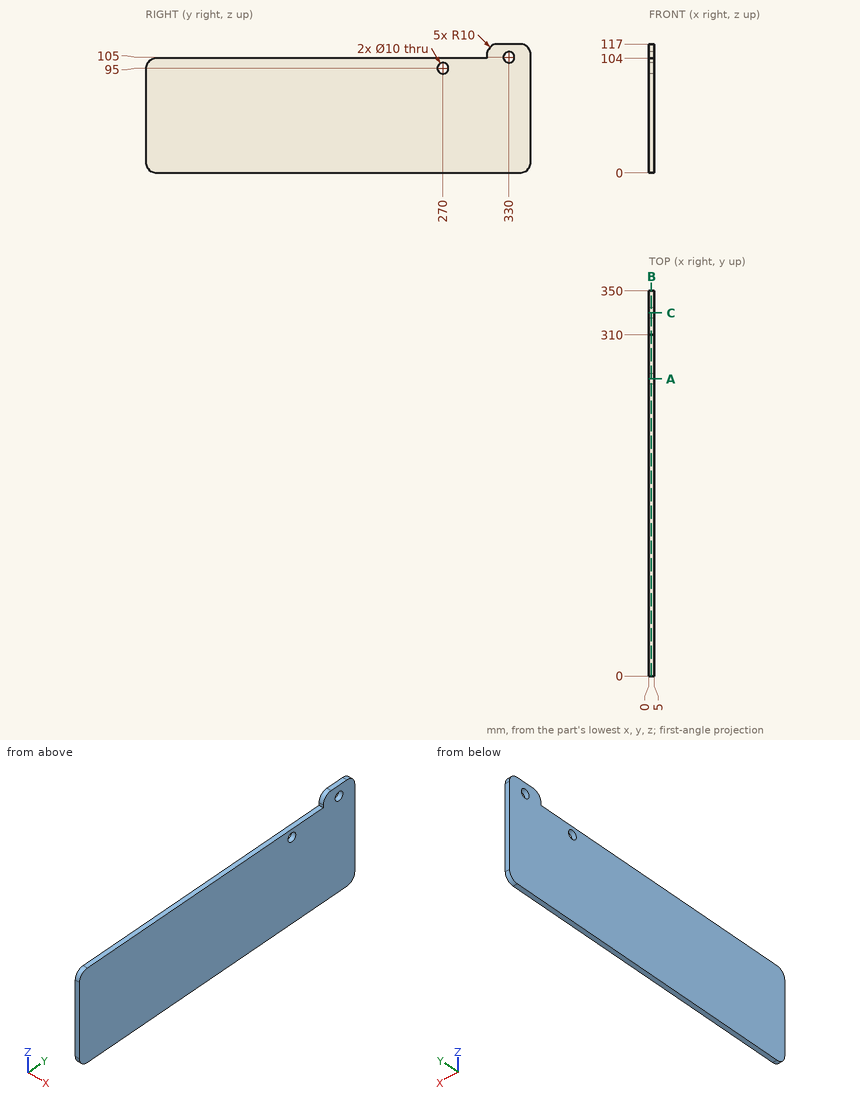
The drawing under review shows one solid part. Ordinate dimensions are in mm from its lowest x, y, z. Give positions to 0.01 mm unless a question says otherwise; leave off trailing zeros. Order: outer loops, then holes, each group sorted by start corner. A loop starts at its lowest first (then second) coordinate and runs counter-clockwise, first axis right, second up. Notation, with made-up numbers: M 37,-9 L 57,-9 A31 ccw 57,20 Z; hole C 50,-25.5 d2. An arc over 180 degrees is marked long. Answer in a Markdown table with one row per item. Add a question column.
1. Add section B-B on x = 2.25. State the section outline as (y, z) points.
2. To check wall thickness, follow line 1 along Z through (x, y) = (3.95, 330); line 2 along Z through (x, y) = (2.7, 173); line 3 along Y through (x, z) = (3.5, 102.5). State the ranges of each line that lie inside material, in increasing order.
3. Add section A-A on y = 270. State the section outline as (x, z) points, plus the area to 3 significant figures.
4. For pin 1 Ø2 at (x, y) = (4, 246) entering from +Z; pin 2 Ø2.5 at (x, z) = (3.5, 105.5) entering from -Y, all flat-tipped, find the tip position at first contact; note any pin that passes through.
5. Add section C-C on y = 330. State the section outline as (x, z) points, plus the area to 3 significant figures.
The answers:
| question | item | result |
|---|---|---|
| 1 | outline | M 0,10 A10 ccw 10,0 L 340,0 A10 ccw 350,10 L 350,107 A10 ccw 340,117 L 320,117 A10 ccw 310,107 L 310,104 L 10,104 A10 ccw 0,94 Z; hole C 270,95 d10; hole C 330,105 d10 |
| 2 | line 1 | 0 to 100, 110 to 117 |
| 2 | line 2 | 0 to 104 |
| 2 | line 3 | 4.73 to 325.67, 334.33 to 350 |
| 3 | outline | M 0,0 L 5,0 L 5,90 L 0,90 Z; M 0,100 L 5,100 L 5,104 L 0,104 Z |
| 3 | area | 470 mm2 |
| 4 | pin 1 | z = 104 |
| 4 | pin 2 | y = 310 |
| 5 | outline | M 0,0 L 5,0 L 5,100 L 0,100 Z; M 0,110 L 5,110 L 5,117 L 0,117 Z |
| 5 | area | 535 mm2 |
